Build history of the part. All positions in model axes, mm. A direction names the side the tool comes from. Coordinates: 2 decimals unless noted, no trailing zeros. Order: outer loops, then holes, each group sorted by start corner. A loop starts at its lowest first (then second) coordinate and runs counter-clockwise, first axis right, second up. Notation, with made-up numbers: (57, 37.25) - (74, 37.25) arc R25 cw to (74, 52.25) - close; hole circle Ø1 at (32.25, 32). An arc over 180 degrees is marked (long way). One line per item, written item: value.
from build123d import *

# Parameters (mm, degrees)
F0_W     = 76.2
F0_H     = 76.2
F1_DEPTH = 76.2
F2_R     = 12.7
F3_DEPTH = 25.4
F4_W     = 25.4
F4_H     = 25.4
F5_DEPTH = 25.4
F6_R     = 12.7
F7_DEPTH = 25.4


with BuildPart() as f1:
    # F0 (on Front) → F1 (new body)
    with BuildSketch(Plane.XZ):
        with Locations((-38.1, 38.1)):
            Rectangle(F0_W, F0_H)
    extrude(amount=F1_DEPTH)

    # F2 (on face) → F3 (cut)
    with BuildSketch(Plane.XY.offset(76.2)):
        with Locations((-38.1, -38.1)):
            Circle(F2_R)
    extrude(amount=-F3_DEPTH, mode=Mode.SUBTRACT)

    # F4 (on face) → F5 (join)
    with BuildSketch(Plane.YZ):
        with Locations((-38.1, 43.252745)):
            Rectangle(F4_W, F4_H)
    extrude(amount=F5_DEPTH)

    # F6 (on face) → F7 (join)
    with BuildSketch(Plane(origin=(0, 0, 0), x_dir=(-1, 0, 0), z_dir=(0, 1, 0))):
        with Locations((38.1, 38.1)):
            Circle(F6_R)
    extrude(amount=F7_DEPTH)


solid = f1.part
1. Band-saw the part on B-B, the plane x = -38.1. Give the cut face in (y, z).
Values found:
outline: (-76.2, 0) - (0, 0) - (0, 25.4) - (25.4, 25.4) - (25.4, 50.8) - (0, 50.8) - (0, 76.2) - (-25.4, 76.2) - (-25.4, 50.8) - (-50.8, 50.8) - (-50.8, 76.2) - (-76.2, 76.2) - close
2. Band-saw the part on D-D, the plane z = 20. Give the cut face in (x, y).
Values found:
outline: (-76.2, -76.2) - (0, -76.2) - (0, 0) - (-76.2, 0) - close
3. Probe line 1 along Y through (x, z) = (-38.1, 59.25); line 2 along Y through (x, z) = (-25, 55.5); line 3 along X through (y, z) = (-30, 63.5). List the from-to ranges inside material, lowest first.
Values found:
line 1: y = -76.2 to -50.8, -25.4 to 0
line 2: y = -76.2 to 0
line 3: x = -76.2 to -47.88, -28.32 to 0
4. Two-plate mould, pull along X, no slides. Class faces 1 (the face through (-76.2, -38, 38)), 2 (the face through (13, -38, 30.553)), 3 (the face through (-38, -38, 50.8)): pulls with the +X half, pulls with the -X half, needs draft (parallel to the pull), parting line crosses it, or undercut.
Values found:
face 1: pulls with the -X half
face 2: needs draft
face 3: undercut
5. Band-saw the part on C-C, the plane z = 66. Give the cut face in (x, y), and give its area (3 significant figures).
Values found:
outline: (-76.2, -76.2) - (0, -76.2) - (0, 0) - (-76.2, 0) - close; hole circle Ø25.4 at (-38.1, -38.1)
area: 5,300 mm2
6. Flat gauge pins, fed straight in: P1, Ø7.5, axis at x = 15, z = 47.5, coming from the +Y side; P2, Ø8, axis at x = -17.5, z = 55.5, coming from the +Y side; P3, Ø12, axis at x = 9.5, z = 35.5, coming from the -Y side. Where does each tip first touch, or does it go through?
Values found:
P1: stops at y = -25.4
P2: stops at y = 0
P3: stops at y = -50.8
7. 3-axis set-ups, long thin cutter, end or side, ignore diameter. For faces 4 (the face through (13, -38, 55.953)), 5 (the face through (-48.2, -45.8, 63.7)), 6 (the face through (13, -25.4, 43)), 7 (the face through (-56, 0, 39)): which of +Z, -Z, +X, -X, +Y, -Y reach the whole face in a straight line?
Values found:
face 4: +Z, +X, +Y, -Y
face 5: +Z
face 6: +Z, -Z, +X, +Y
face 7: +Y
8. Band-saw the part on A-A, the plane y = -38.1. Give the cut face in (x, z).
Values found:
outline: (-76.2, 0) - (0, 0) - (0, 30.55) - (25.4, 30.55) - (25.4, 55.95) - (0, 55.95) - (0, 76.2) - (-25.4, 76.2) - (-25.4, 50.8) - (-50.8, 50.8) - (-50.8, 76.2) - (-76.2, 76.2) - close
